Autodesk Inventor part; units mm, degrees
ref_plane "YZ Plane" through (0, 0, 0) normal (1, 0, 0) x (0, 1, 0)
ref_plane "XZ Plane" through (0, 0, 0) normal (0, 1, 0) x (-1, 0, 0)
ref_plane "XY Plane" through (0, 0, 0) normal (0, 0, 1) x (1, 0, 0)
sketch "草圖1" plane through (0, 0, 0) normal (0, 0, 1) x (1, 0, 0)
  line L0 (0, 0) -> (40, 0)
  line L1 (40, 0) -> (40, 50)
  line L2 (40, 50) -> (0, 50)
  line L3 (0, 50) -> (0, 0)
  circle A0 centre (20, 30) radius 10
  dimension "d0" = 20
  dimension "d1" = 40
  dimension "d2" = 50
  dimension "d3" = 20
  dimension "d4" = 30
extrude "擠出1" add sketch "草圖1" along normal mid plane 20
sketch "草圖2" plane through (0, 0, 0) normal (0, 0, 1) x (1, 0, 0)
  line L0 (40, 0) -> (40, 50)
  line L1 (40, 30) -> (80, 30)
  line L2 (80, 30) -> (80, 20)
  line L3 (80, 20) -> (40, 20)
  line L4 (40, 20) -> (40, 30)
  line L5 (0, 0) -> (40, 0)
  dimension "d7" = 20
  dimension "d8" = 10
  dimension "d9" = 40
extrude "擠出2" add sketch "草圖2" along normal mid plane 40
fillet "圓角1" radius 20 2 edges at (80, 25, -20) (80, 25, 20)
fillet "圓角2" radius 10 2 edges at (40, 30, 0) (40, 20, 0)
fillet "圓角3" radius 10 2 edges at (0, 50, 0) (0, 0, 0)
sketch "草圖3" plane through (40, 30, 20) normal (0, 1, 0) x (1, 0, 0)
  arc A0 (20, 0) -> (20, 40) centre (20, 20) ccw
  point P0 (-40, 20)
hole "孔1" at (60, 30, 0) direction (0, -1, 0) diameter 20 end through all
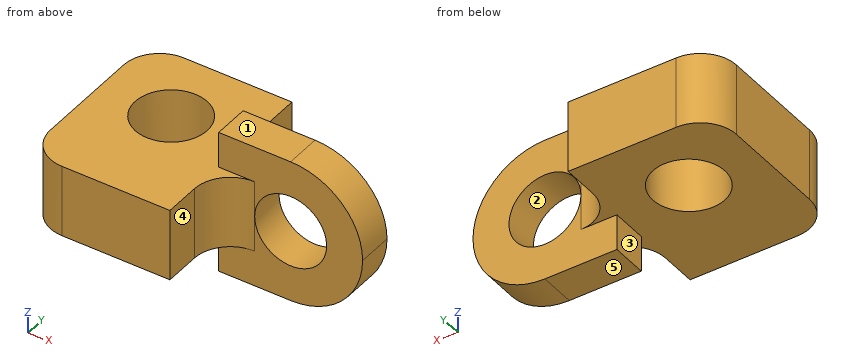
Could you check a few things on this model? Use its own coordinates, in mm. Face numbers are marked on the shaded views. A direction names the side the tool comes from. Coordinates: 2 decimals unless noted, no trailing zeros. Write each loop counter-clockwise with the first axis right and the second up, starting at its lowest first coordinate (ties: lowest second). Pieces come first, ordered by that corner, then holes. Notation, with made-up numbers: (44.25, 50.25) - (88.25, 50.25) arc R26 ccw to (88.25, 72.25) - close; hole circle Ø7 at (-33, 64.25). An arc over 180 degrees is marked (long way). Use a Markdown table: item, result.
Q1. Imagine slicing it at B-B (z = 5). List the corners of the cut face in (x, y) for me.
Geometry check:
| item | result |
|---|---|
| outline | (0, 10) arc R10 ccw to (10, 0) - (40, 0) - (40, 10) arc R10 cw to (50, 20) - (51.34, 20) - (51.34, 30) - (50, 30) arc R10 cw to (40, 40) - (40, 50) - (10, 50) arc R10 ccw to (0, 40) - close; (68.66, 20) - (79.37, 20) - (79.37, 30) - (68.66, 30) - close; hole circle Ø20 at (20, 30) |
Q2. Imagine slicing it at A-A (x = 20). List the corners of the cut face in (y, z) for me.
Geometry check:
| item | result |
|---|---|
| outline | (0, -10) - (20, -10) - (20, 10) - (0, 10) - close; (40, -10) - (50, -10) - (50, 10) - (40, 10) - close |
Q3. Please list where these lines run through material, in increasing order: L1, parallel to Y at x = 20, z = -5; L2, parallel to Z at x = 60, y = 27; L3, parallel to X at y = 24, z = 0.
Geometry check:
| item | result |
|---|---|
| L1 | y = 0 to 20, 40 to 50 |
| L2 | z = -20 to -10, 10 to 20 |
| L3 | x = 0 to 12, 28 to 50, 70 to 80 |
Q4. Thinking about a two-plate mould opening in Z: for the marked faces 1, 2 and 3, which applies, +Z half, -Z half, draft (parallel to the pull), parting line (faces both ways), or undercut?
Geometry check:
| item | result |
|---|---|
| face 1 | +Z half |
| face 2 | undercut |
| face 3 | draft |
Q5. Imagine slicing it at C-C (z = -9). List the corners of the cut face in (x, y) for me, and give its area (3 significant figures).
Geometry check:
| item | result |
|---|---|
| outline | (0, 10) arc R10 ccw to (10, 0) - (40, 0) - (40, 10) arc R10 cw to (50, 20) - (55.64, 20) - (55.64, 30) - (50, 30) arc R10 cw to (40, 40) - (40, 50) - (10, 50) arc R10 ccw to (0, 40) - close; (64.36, 20) - (77.86, 20) - (77.86, 30) - (64.36, 30) - close; hole circle Ø20 at (20, 30) |
| area | 1,980 mm2 |
Q6. I'm going to push flat-ended pins straight in: pin 1 Ø3 at (y, z) = (27, -17) entering from -X; pin 2 Ø12 at (x, z) = (60, 0) entering from -Y; pin 3 Ø12 at (x, z) = (68.5, 1.5) entering from -Y; pin 4 Ø15 at (x, y) = (19, 21) entering from -Z. Where does each tip first touch, or does it pass through?
Geometry check:
| item | result |
|---|---|
| pin 1 | stops at x = 40 |
| pin 2 | passes through |
| pin 3 | stops at y = 20 |
| pin 4 | stops at z = -10 |
Q7. Which directions (+Z, -Z, +X, -X, +Y, -Y) give clear straight access to the entire face, cutting with the end or side of a thin tool? Please do the marked faces 4 and 5.
Geometry check:
| item | result |
|---|---|
| face 4 | +Z, -Z, +X, -Y |
| face 5 | -Z, +X, -X, +Y, -Y |
Q8. Imagine slicing it at D-D (x = 42.5). List the corners of the cut face in (y, z) for me.
Geometry check:
| item | result |
|---|---|
| outline | (16.61, -10) - (20, -10) - (20, -20) - (30, -20) - (30, -10) - (33.39, -10) - (33.39, 10) - (30, 10) - (30, 20) - (20, 20) - (20, 10) - (16.61, 10) - close |
